Geometry check sheet. Reference: the model listing, model coordinates, mm. Face numbers are marked on the shaded views. A direction names the side the tool comes from. Coordinates: 2 decimals unless noted, no trailing zeros. Loops run counter-clockwise (first coordinate to the right, second up) from the corner with the lowest first, then second, coordinate; pieces in that order, holes last.
from build123d import *

# Parameters (mm, degrees)
SKETCH1_W               = 63.5
SKETCH1_H               = 57.15
BOSS_EXTRUDE1_DEPTH     = 38.1
SKETCH2_W               = 50.8
SKETCH2_H               = 12.7
CUT_EXTRUDE1_DEPTH      = 94.541341128
SKETCH3_W               = 63.5
SKETCH3_H               = 25.4
CUT_EXTRUDE2_DEPTH      = 38.1
FILLET3_R               = 6.35
FILLET4_R               = 6.35
SKETCH4_R               = 3.252730628
SKETCH4_R_2             = 3.379495502
SKETCH4_R_3             = 8.895504244
CUT_EXTRUDE3_DEPTH      = 94.541341128
CHAMFER1_SIZE           = 0.762
CHAMFER2_SIZE           = 0.762
CUT_EXTRUDE5_DEPTH      = 92.139645599
CUT_EXTRUDE5_DEPTH_BACK = 92.139645599
CHAMFER3_SIZE           = 0.762
CHAMFER3_SIZE_2         = 1.762810924


# Some blends are built 0.0001 mm under size
with BuildPart() as part:
    # Sketch1 → Boss-Extrude1 (new body)
    with BuildSketch(Plane.XY):
        with Locations((31.75, 28.575)):
            Rectangle(SKETCH1_W, SKETCH1_H)
    extrude(amount=BOSS_EXTRUDE1_DEPTH)

    # Sketch2 → Cut-Extrude1 (cut, through all)
    with BuildSketch(Plane(origin=(0, 0, 0), x_dir=(-1, 0, 0), z_dir=(0, 0, -1))):
        with Locations((-31.75, 6.35)):
            Rectangle(SKETCH2_W, SKETCH2_H)
    extrude(amount=-CUT_EXTRUDE1_DEPTH, mode=Mode.SUBTRACT)

    # Sketch3 → Cut-Extrude2 (cut)
    with BuildSketch(Plane(origin=(0, 57.15, 0), x_dir=(1, 0, 0), z_dir=(0, 1, 0))):
        with Locations((31.75, -19.05)):
            Rectangle(SKETCH3_W, SKETCH3_H)
    extrude(amount=-CUT_EXTRUDE2_DEPTH, mode=Mode.SUBTRACT)

    # Fillet3
    fillet3_edges = [part.edges().sort_by_distance(p)[0] for p in [
        (31.75, 57.15, 38.1),
    ]]
    fillet(fillet3_edges, radius=FILLET3_R - 0.0001)  # a hair under: the kernel refuses the full size

    # Fillet4
    fillet4_edges = [part.edges().sort_by_distance(p)[0] for p in [
        (31.75, 57.15, 0),
    ]]
    fillet(fillet4_edges, radius=FILLET4_R - 0.0001)  # a hair under: the kernel refuses the full size

    # Sketch4 → Cut-Extrude3 (cut, through all)
    with BuildSketch(Plane(origin=(0, 0, 0), x_dir=(-1, 0, 0), z_dir=(0, 0, -1))):
        with Locations((-57.15, 35.819311932)):
            Circle(SKETCH4_R)
        with Locations((-6.35, 35.819311932)):
            Circle(SKETCH4_R_2)
        with Locations((-31.75, 35.819311932)):
            Circle(SKETCH4_R_3)
    extrude(amount=-CUT_EXTRUDE3_DEPTH, mode=Mode.SUBTRACT)

    # Chamfer1
    chamfer1_edges = [part.edges().sort_by_distance(p)[0] for p in [
        (63.5, 55.29015735, 1.85984265),
        (63.5, 25.40005, 0),
    ]]
    chamfer(chamfer1_edges, length=CHAMFER1_SIZE)

    # Chamfer2
    chamfer2_edges = [part.edges().sort_by_distance(p)[0] for p in [
        (0, 25.40005, 38.1),
        (63.5, 55.29015735, 36.24015735),
        (0, 55.29015735, 36.24015735),
        (0, 25.40005, 0),
        (0, 55.29015735, 1.85984265),
        (63.5, 25.40005, 38.1),
    ]]
    chamfer(chamfer2_edges, length=CHAMFER2_SIZE)

    # Sketch5 → Cut-Extrude5 (cut, two sides: drawn at the far end of the back side and taken through both)
    with BuildSketch(Plane(origin=(0, 0, 31.75), x_dir=(-1, 0, 0), z_dir=(0, 0, -1)).offset(-CUT_EXTRUDE5_DEPTH_BACK)):
        with BuildLine():
            Line((152.450199575, -35.171760157), (1.839159199, 45.87092885))
            ThreePointArc((1.839159199, 45.87092885), (-32.809317684, 54.236506182), (-67.098653648, 44.502993274))
            Line((-67.098653648, 44.502993274), (-214.376135409, -42.450708722))
            Line((-214.376135409, -42.450708722), (-221.162348462, 299.543968154))
            Line((-221.162348462, 299.543968154), (145.663986523, 306.822916719))
            Line((145.663986523, 306.822916719), (152.450199575, -35.171760157))
        make_face()
    extrude(amount=CUT_EXTRUDE5_DEPTH + CUT_EXTRUDE5_DEPTH_BACK, mode=Mode.SUBTRACT)

    # Chamfer3
    # the kernel refuses this chamfer: 1.762810924, 1.706340641, 0.762 mm, written as the material it takes off along each edge
    with BuildSketch(Plane(origin=(0, 46.825825111, -3.52035895), x_dir=(0.8994074011398961, 0.43711134368119303, 0), z_dir=(0, 0, 1))) as chamfer3_piece_1:
        with BuildLine():
            Line((1.648294394, 0), (-CHAMFER3_SIZE * 0.437111343681, -CHAMFER3_SIZE * 0.89940740114))
            Line((-CHAMFER3_SIZE * 0.437111343681, -CHAMFER3_SIZE * 0.89940740114), (0, 0))
            ThreePointArc((0, 0), (0.856396227, 0.004831664), (1.648294394, 0))
        make_face()
    extrude(amount=14.152717899, mode=Mode.SUBTRACT)
    with BuildSketch(Plane(origin=(0, 46.825825111, 27.46764105), x_dir=(0, -1, 0), z_dir=(0, 0, 1))) as chamfer3_piece_2:
        with BuildLine():
            Line((CHAMFER3_SIZE, 0), (-0.720488177, 1.482488177))
            ThreePointArc((-0.720488177, 1.482488177), (-0.37868614, 0.76813713), (0, 0))
            Line((0, 0), (CHAMFER3_SIZE, 0))
        make_face()
    extrude(amount=14.152717899, mode=Mode.SUBTRACT)
    with BuildSketch(Plane(origin=(63.5, 46.487927277, -3.813189181), x_dir=(-0.8918533135709217, 0.4523247363040928, 0), z_dir=(0, 0, 1))) as chamfer3_piece_3:
        with BuildLine():
            Line((0.757918605, 0), (-CHAMFER3_SIZE_2 * 0.452324736297, CHAMFER3_SIZE_2 * 0.891853313556))
            Line((-CHAMFER3_SIZE_2 * 0.452324736297, CHAMFER3_SIZE_2 * 0.891853313556), (0, 0))
            ThreePointArc((0, 0), (0.403745747, -0.001018742), (0.757918605, 0))
        make_face()
    extrude(amount=14.738378362, mode=Mode.SUBTRACT)
    with BuildSketch(Plane(origin=(63.5, 46.487927277, 27.174810819), x_dir=(0, -1, 0), z_dir=(0, 0, 1))) as chamfer3_piece_4:
        with BuildLine():
            Line((CHAMFER3_SIZE_2, 0), (-0.342825333, -0.675952219))
            ThreePointArc((-0.342825333, -0.675952219), (-0.183532757, -0.35962118), (0, 0))
            Line((0, 0), (CHAMFER3_SIZE_2, 0))
        make_face()
    extrude(amount=14.738378362, mode=Mode.SUBTRACT)


solid = part.part
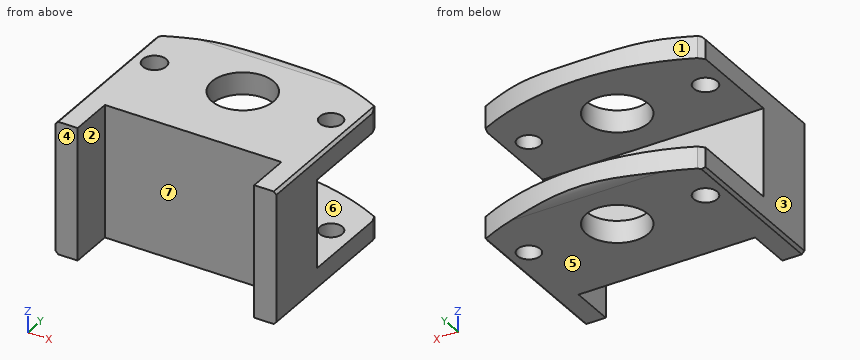
1) Section check C-C on x = 31.75. Record the cut outline in (y, z).
Data:
outline: (12.7, 0) - (26.92, 0) - (26.92, 6.35) - (19.05, 6.35) - (19.05, 31.75) - (26.92, 31.75) - (26.92, 38.1) - (12.7, 38.1) - close; (44.71, 0) - (50.8, 0) arc R6.35 ccw to (54.25, 1.02) - (54.25, 6.35) - (44.71, 6.35) - close; (44.71, 31.75) - (54.25, 31.75) - (54.25, 37.08) arc R6.35 ccw to (50.8, 38.1) - (44.71, 38.1) - close
2) Access from +Z, -Z, +X, -X, +Y, -Y to the whole of each face (thin tool, end or side, straight path). Record for the marked faces 5, 6 and 7.
Data:
face 5: -Z, +X, -X, +Y, -Y
face 6: +X, -X, +Y
face 7: +Z, -Z, -Y
3) Section check B-B on z = 17.5. Record the cut outline in (x, y).
Data:
outline: (0, 0) - (6.35, 0) - (6.35, 12.7) - (57.15, 12.7) - (57.15, 0) - (63.5, 0) - (63.5, 19.05) - (0, 19.05) - close
4) Material ranges on probe 1 along Z at (x, y) = (19, 46.5); probe 2 along X at (y, z) = (8.5, 14), recorded low to high.
Data:
probe 1: z = 0 to 6.35, 31.75 to 38.1
probe 2: x = 0 to 6.35, 57.15 to 63.5
5) Section check A-A on y = 8. Record the cut outline in (x, z), and give its area (3 significant figures).
Data:
outline: (0, 0.76) - (0.76, 0) - (6.35, 0) - (6.35, 38.1) - (0.76, 38.1) - (0, 37.34) - close; (57.15, 0) - (62.74, 0) - (63.5, 0.76) - (63.5, 37.34) - (62.74, 38.1) - (57.15, 38.1) - close
area: 483 mm2
6) Section check D-D on y = 30.5. Record the cut outline in (x, z).
Data:
outline: (0, 0.76) - (0.76, 0) - (24.62, 0) - (24.62, 6.35) - (0, 6.35) - close; (0, 31.75) - (24.62, 31.75) - (24.62, 38.1) - (0.76, 38.1) - (0, 37.34) - close; (38.88, 0) - (62.74, 0) - (63.5, 0.76) - (63.5, 6.35) - (38.88, 6.35) - close; (38.88, 31.75) - (63.5, 31.75) - (63.5, 37.34) - (62.74, 38.1) - (38.88, 38.1) - close
7) Depth check by flat-ended pin: pin 1 (6 mm diameter, centred on y = 32.5, z = 33, fed in from -X); pin 2 (20.5 mm diameter, centred on x = 32.5, z = 17.5, fed in from +Y); pin 3 (10 mm diameter, centred on x = 24.5, z = 9, fed in from -Y). Enter the tip coordinate at first touch or a pass-through.
Data:
pin 1: stops at x = 0
pin 2: stops at y = 19.05
pin 3: stops at y = 12.7
8) Mould release check, pull along X, two halves, no side actions. Record for the marked faces 1, 2, 3 and 4: +X half, -X half, draft (parallel to the pull), parting line (faces both ways), or undercut.
Data:
face 1: parting line
face 2: undercut
face 3: -X half
face 4: draft
